Verification items for the finished model (mm, model axes). A direction names the side the tool comes from. Give positions to 0.01 mm unless a question says otherwise; leave off trailing zeros. Order: outer loops, then holes, each group sorted by start corner. A loop starts at its lowest first (then second) coordinate and runs counter-clockwise, first axis right, second up. Notation, with made-up numbers: M -22,-28 L 10,-28 A32 cw 10,5 Z; hole C 0,31 d8. An arc over 180 degrees is marked long. Answer as a JSON object with one key per item and string values.
```python
from build123d import *


with BuildPart() as f1:
    # F0 (on Right) → F1 (revolve)
    with BuildSketch(Plane.YZ):
        with BuildLine():
            Line((0.4572, 6.230392), (0, 6.230392))
            Line((0, 6.230392), (0, 3.5))
            Line((0, 3.5), (35.306, 3.5))
            Line((35.306, 3.5), (35.306, 4.836943))
            Line((35.306, 4.836943), (31.528782, 5.541712))
            Line((31.528782, 5.541712), (31.528782, 4.836943))
            Line((31.528782, 4.836943), (27.751564, 5.541712))
            Line((27.751564, 5.541712), (27.751564, 4.836943))
            Line((27.751564, 4.836943), (23.974346, 5.541712))
            Line((23.974346, 5.541712), (23.974346, 4.952836))
            Line((23.974346, 4.952836), (18.796, 5.541712))
            Line((18.796, 5.541712), (18.796, 7.62))
            Line((18.796, 7.62), (16.51, 7.62))
            Line((16.51, 7.62), (16.51, 4.529946))
            Line((16.51, 4.529946), (11.654421, 4.529946))
            Line((11.654421, 4.529946), (11.654421, 6.230392))
            Line((11.654421, 6.230392), (1.145791, 6.230392))
            ThreePointArc((1.145791, 6.230392), (0.801495, 6.446617), (0.4572, 6.230392))
        make_face()
    revolve(axis=Axis((0, 43.56328, 0), (0, 1, 0)))


solid = f1.part
```
Q1. Material ranges on L1, parallel to Y at x = -0.5, z = -6; L2, parallel to X at y = 15.5, z = 0; L3, parallel to Y at x = -4, z = 5.25, recorded low to high.
Resolved:
{"L1": "y = 0 to 11.65, 16.51 to 18.8", "L2": "x = -4.53 to -3.5, 3.5 to 4.53", "L3": "y = 16.51 to 18.8"}
Q2. Release check for a two-part mould opening along X. For faces 1 (the face through (-1.341, 17.9, 3.233)), 2 (the face through (-5.063, 21.924, -1.124)), 3 (the face through (-6, 18.796, -1)) record: +X half, -X half, draft (parallel to the pull), parting line (faces both ways), or undercut.
Resolved:
{"face 1": "undercut", "face 2": "parting line", "face 3": "draft"}
Q3. Section check A-A on y = 17.5. Record the cut outline in (x, z), then the cut area to 3 significant figures.
Resolved:
{"outline": "C 0,0 d15.24; hole C 0,0 d7", "area": "144 mm²"}
Q4. Gauge pin test, flat ends, axial feed: pin 1 Ø5 at (x, y) = (-1, 3.5) entering from -Z; pin 2 Ø6 at (x, y) = (0.5, 8) entering from +Z; pin 3 Ø3 at (x, y) = (-3, 22) entering from +Z. Record the tip position at first contact, or that the pin passes through.
Resolved:
{"pin 1": "stops at z = -6.34", "pin 2": "stops at z = 6.23", "pin 3": "stops at z = 4.99"}
Q5. Tool access check on faces 4 (the face through (1.513, 34.23, 4.805)), 5 (the face through (-5, 11.654, 0)), 6 (the face through (4.2, 0.2, -4.6)). Record the directions out of +Z, -Z, +X, -X, +Y, -Y that give a thin tool (end or side, any length) a straight path to the whole face; none if there is none.
Resolved:
{"face 4": "+Y", "face 5": "none", "face 6": "-Y"}
